```python
from build123d import *

# Parameters (mm, degrees)
BOSS_EXTRU_1_DEPTH      = 216
ENL_V_MAT_EXTRU_1_DEPTH = 41
ENL_V_MAT_EXTRU_2_DEPTH = 41


with BuildPart() as part:
    # Esquisse1 → Boss.-Extru.1 (new body)
    with BuildSketch(Plane(origin=(0, 0, 0), x_dir=(0, 0, -1), z_dir=(1, 0, 0))):
        Polygon((0, 0), (-40, 0), (-40, -17), (-17, -17), (-17, -40), (0, -40), align=None)
    extrude(amount=BOSS_EXTRU_1_DEPTH)

    # Esquisse2 → Enlèv. mat.-Extru.1 (cut, through all)
    with BuildSketch(Plane(origin=(0, 0, 0), x_dir=(1, 0, 0), z_dir=(0, 1, 0))):
        Polygon((216, 0), (176, -40), (216, -40), align=None)
        Polygon((0, 0), (0, -40), (40, -40), align=None)
    extrude(amount=-ENL_V_MAT_EXTRU_1_DEPTH, mode=Mode.SUBTRACT)

    # Esquisse3 → Enlèv. mat.-Extru.2 (cut, through all)
    with BuildSketch(Plane(origin=(0, 0, 0), x_dir=(-1, 0, 0), z_dir=(0, 0, -1))):
        Polygon((-216, 0), (-176, -40), (-216, -40), align=None)
        Polygon((-40, -40), (0, -40), (0, 0), align=None)
    extrude(amount=-ENL_V_MAT_EXTRU_2_DEPTH, mode=Mode.SUBTRACT)


solid = part.part
```
For this review, take the finished solid that the model builds, in its own axes (mm). A direction names the side the tool comes from. Round coordinates to 2 decimals unless told otherwise and drop trailing zeros. Order: outer loops, then holes, each group sorted by start corner. A loop starts at its lowest first (then second) coordinate and runs counter-clockwise, first axis right, second up.
Q1. We need section B-B, the plane x = 34.5. Give the boundary of the cut face in (y, z), plus the area to 3 significant figures.
Findings below:
outline: (-34.5, 0) - (0, 0) - (0, 34.5) - (-17, 34.5) - (-17, 17) - (-34.5, 17) - close
area: 884 mm2
Q2. Wall thickness on line 1 (Y direction, x = 22.5, z = 21.5); line 2 (X direction, y = -1.5, z = 10.5); line 3 (Z direction, x = 85, y = -23.5): over which ranges is each line inside the solid? List them lowest first.
Findings below:
line 1: y = -17 to 0
line 2: x = 10.5 to 205.5
line 3: z = 0 to 17
Q3. We need section C-C, the plane y = -23. Give the boundary of the cut face in (x, z).
Findings below:
outline: (23, 0) - (193, 0) - (193, 17) - (23, 17) - close
Q4. Insertion check: P1, Ø1, axis at y = -5.5, z = 25.5, coming from the +X side; P2, Ø1.5, axis at x = 57.5, y = -23, coming from the +Z side; P3, Ø7, axis at x = 129.5, z = 30, coming from the -Y side. Each pin has a flat end and moves straight along its axis. Give the tip position at first contact, or say it passes through.
Findings below:
P1: stops at x = 191
P2: stops at z = 17
P3: stops at y = -17
Q5. Machinability: for faces 1 (the flat face through (106, -20, 0)), 2 (the flat face through (107, -28, 17)), which of the approach directions +Z, -Z, +X, -X, +Y, -Y give a long, thin tool a straight path to every point of the face, cutting with its end or side? Answer none if there is none.
Findings below:
face 1: -Z, +X, -X, +Y, -Y
face 2: +Z, +X, -X, -Y
Q6. We need section D-D, the plane z = 23.5. Give the boundary of the cut face in (x, y), plus the area to 3 significant figures.
Findings below:
outline: (23.5, -17) - (192.5, -17) - (192.5, 0) - (23.5, 0) - close
area: 2,870 mm2
Q7. We need section A-A, the plane z = 14.5. Give the boundary of the cut face in (x, y).
Findings below:
outline: (14.5, -14.5) - (40, -40) - (176, -40) - (201.5, -14.5) - (201.5, 0) - (14.5, 0) - close
